Autodesk Inventor part; units mm, degrees
ref_plane "IDS_WORKPLANE{1}" through (-2.8448, 0, 0) normal (1, 0, 0) x (0, 0, -1)
ref_plane "Work Plane2" through (-1.4224, 0, 0) normal (0, 0, -1) x (1, 0, 0)
ref_plane "YZ Plane" through (0, 0, 0) normal (1, 0, 0) x (0, 1, 0)
sketch "Sketch1" plane through (0, 0, 0) normal (0, 0, 1) x (1, 0, 0)
  line L0 (-2.8448, 0) -> (9.525, 0)
  line L1 (9.525, 0) -> (9.525, 1.4224)
  line L2 (9.525, 1.4224) -> (0, 1.4224)
  line L3 (0, 1.4224) -> (0, 2.3241)
  line L4 (-7.3162, 0) -> (16.036, 0)
  line L5 (0, -0.4648) -> (0, 2.7889)
  line L6 (0, 2.3241) -> (-2.8448, 2.3241)
  line L7 (-2.8448, 0) -> (-2.8448, 2.3241)
  arc A0 (-1.1734, 0) -> (-1.5494, 1.4034) centre (-3.9802, 0) ccw
  line L8 (-2.8448, 1.4034) -> (-1.5494, 1.4034)
  line L9 (12.7, 1.4224) -> (0, 1.4224) construction
  dimension "d0" = 9.525
  dimension "d1" = 2.8448
  dimension "d2" = 2.8448
  dimension "d5" = 4.6482
  dimension "d13" = 2.8068
  dimension "d14" = 2.8068
  dimension "d15" = 1.2954
revolve "Body" add sketch "Sketch1" angle 360 about axis through (-2.8448, 0, 0) along (1, 0, 0) contours A0 L8 L7 L6 L3 L5 L0 | L5 L2 L1 L0
ref_plane "IDS_WORKPLANE{1}" through (-2.8448, 0, 0) normal (1, 0, 0) x (0, 0, -1)
sketch "Sketch2" plane through (-2.8448, 0, 0) normal (1, 0, 0) x (0, 0, -1)
  line L0 (0, -3.6027) -> (0, 5.3473)
  line L1 (5.6384, 0) -> (-3.6512, 0)
  circle A0 centre (0, 0) radius 2.3241
  line L2 (1.3655, 0.3238) -> (1.1714, 0.3239)
  line L3 (0, 0) -> (1.3655, 0.3238) construction
  line L4 (0, 0) -> (4.3113, 4.0687) construction
  line L5 (0, 0) -> (0.4023, 1.3445) construction
  line L6 (0, 0) -> (0.7017, 1.2154) construction
  line L7 (0.4023, 1.3445) -> (0.3053, 1.1764)
  line L8 (0.9632, 1.0207) -> (0.8662, 0.8526)
  line L9 (0, 0) -> (0.9632, 1.0207) construction
  arc A1 (1.2154, 0) -> (1.1714, 0.3239) centre (0, 0) ccw
  arc A2 (0.8662, 0.8526) -> (0.3053, 1.1764) centre (0, 0) ccw
  arc A3 (1.4034, 0) -> (1.3655, 0.3238) centre (0, 0) ccw
  arc A4 (0.9632, 1.0207) -> (0.4023, 1.3445) centre (0, 0) ccw
  arc A5 (1.3655, 0.3238) -> (0.8276, 1.1334) centre (0, 0) ccw construction
  arc A6 (1.1714, 0.3239) -> (0.8662, 0.8526) centre (0, 0) ccw construction
  line L10 (1.3655, -0.3238) -> (1.1714, -0.3239)
  line L11 (0.4023, -1.3445) -> (0.3053, -1.1764)
  line L12 (0.9632, -1.0207) -> (0.8662, -0.8526)
  arc A7 (1.1714, -0.3239) -> (1.2154, 0) centre (0, 0) ccw
  arc A8 (0.3053, -1.1764) -> (0.8662, -0.8526) centre (0, 0) ccw
  arc A9 (1.3655, -0.3238) -> (1.4034, 0) centre (0, 0) ccw
  arc A10 (0.4023, -1.3445) -> (0.9632, -1.0207) centre (0, 0) ccw
  line L13 (-1.3655, 0.3238) -> (-1.1714, 0.3239)
  line L14 (-0.4023, 1.3445) -> (-0.3053, 1.1764)
  line L15 (-0.9632, 1.0207) -> (-0.8662, 0.8526)
  arc A11 (-1.1714, 0.3239) -> (-1.2154, 0) centre (0, 0) ccw
  arc A12 (-0.3053, 1.1764) -> (-0.8662, 0.8526) centre (0, 0) ccw
  arc A13 (-1.3655, 0.3238) -> (-1.4034, 0) centre (0, 0) ccw
  arc A14 (-0.4023, 1.3445) -> (-0.9632, 1.0207) centre (0, 0) ccw
  line L16 (-0.4023, -1.3445) -> (-0.3053, -1.1764)
  arc A15 (-0.8662, -0.8526) -> (-0.3053, -1.1764) centre (0, 0) ccw
  line L17 (-0.9632, -1.0207) -> (-0.8662, -0.8526)
  arc A16 (-0.9632, -1.0207) -> (-0.4023, -1.3445) centre (0, 0) ccw
  arc A17 (-1.2154, 0) -> (-1.1714, -0.3239) centre (0, 0) ccw
  line L18 (-1.3655, -0.3238) -> (-1.1714, -0.3239)
  arc A18 (-1.4034, 0) -> (-1.3655, -0.3238) centre (0, 0) ccw
  point P0 (0.7017, -1.2154)
  point P1 (-0.7017, 1.2154)
  point P2 (-0.7017, -1.2154)
  dimension "d19" = 0.3239
  dimension "d20" = 0.6477
  dimension "d21" = 33.316
  dimension "d22" = 2.8068
  dimension "d23" = 2.4308
extrude "Slot" add sketch "Sketch2" along normal up to next contours A1 L2 A3 L1 | L1 A9 L10 A7 | A17 L18 A18 L1 | L1 A13 L13 A11 | A4 L8 A2 L7 | L11 A8 L12 A10 | L14 A12 L15 A14 | A16 L17 A15 L16
fillet "Fillet1" radius 0.2286 1 edges at (-2.8448, -2.3241, 0)
thread "Thread"
chamfer "Chamfer1" distance 0.3785 distance2 0.3785 1 edges at (9.525, -1.4224, 0) measured on face at (9.525, -0.2537, -0.5191)
ref_plane "Work Plane2" through (-1.4224, 0, 0) normal (0, 0, -1) x (1, 0, 0)
equation "\"d19\" = 0.5 * SBR"
equation "\"d20\" = SBR"
equation "\"d22\" = 1.1547 * SW"
equation "\"d23\" = SW"
equation "\"d17\" = INTI"
equation "\"d24\" = RR"
equation "\"d6\" = GEL"
equation "\"d9\" = -0.5 * SPD + 0.5 * NND"
equation "\"d10\" = GUL"
equation "\"d0\" = NLG"
equation "\"d1\" = KOH"
equation "\"d2\" = NND"
equation "\"d5\" = KOD"
equation "\"d13\" = 1.1547 * SW"
equation "\"d14\" = 1.1547 * SW"
equation "\"d15\" = INTI"
equation "\"NND\" = 2.8448"
equation "\"NLG\" = 9.525"
equation "\"GEL\" = 7.9375"
equation "\"KOD\" = 4.6482"
equation "\"KOH\" = 2.8448"
equation "\"SPD\" = GD1"
equation "\"GUL\" = 0.37846"
equation "\"SBR\" = 0.6477"
equation "\"INTI\" = 1.2954"
equation "\"d11\" = -KOH"
equation "\"SW\" = 2.43078"
equation "\"d16\" = 1.1547 * SW"
equation "\"d18\" = SW"
equation "\"RR\" = 0.2286"
equation "\"TOA\" = 30deg"
equation "\"GD1\" = 2.08788"
equation "\"THREADDIA\" = 2.8448"
equation "\"BDM\" = NND"
equation "\"GD\" = NND"
equation "\"GAL\" = 1.5875"
equation "\"E0\" = 2.86258"
properties part number "ANSI B18.3 - 4-40 UNC - 0.375, SSHCSI" material "Steel, Mild"
Design review of the part built by this model. Coordinates are the model's own, in mm. A direction names the side the tool comes from. Give positions to 0.01 mm unless a question says otherwise; leave off trailing zeros. Order: outer loops, then holes, each group sorted by start corner. A loop starts at its lowest first (then second) coordinate and runs counter-clockwise, first axis right, second up. Notation, with made-up numbers: (2.25, 74) - (32.25, 74) arc R36 ccw to (32.25, 111) - close; hole circle Ø8 at (-35.75, -6). An arc over 180 degrees is marked (long way). Use a Markdown table: item, result. Add a question column.
(1) Machinability: for faces 5 (the face through (4.51, -0.31, 1.39)), 6 (the face through (9.525, 0, 0)), which of the approach directions +Z, -Z, +X, -X, +Y, -Y give a long, thin tool a straight path to every point of the face, cutting with its end or side? Answer none if there is none.
(2) Add section A-A on x = 0.25. Give the boundary of the cut face in (y, z).
(3) Clearance check with flat-ended pins moving along their axes: P1, Ø1.5, axis at x = 1.5, z = -1.5, coming from the +Y side; P2, Ø1.5, axis at x = 8, z = 2, coming from the -Y side. State where each tip first meets the part, or that it passes through.
(4) Wall thickness on probe 1 along X at (y, z) = (1.75, -1); probe 2 along Y at (x, z) = (1.75, -0.4) (3 decimals); probe 3 along Z at (x, y) = (5, 0.8): over which ranges is each line inside the solid? List them lowest first. Write a range as [from, to].
(5) Mouldability with a two-part tool opening along Z and no side actions: class faces 1 (the face through (-1.33, -0.5, 2.27)), 2 (the face through (-2.188, -1.403, 0.006)), 3 (the face through (-2.845, 0, -1.4)), 4 (the face through (-2.188, 1.403, -0.006)) as +Z half, -Z half, draft (parallel to the pull), parting line (faces both ways), or undercut.
Report:
| question | item | result |
|---|---|---|
| 1 | face 5 | +X |
| 1 | face 6 | +Z, -Z, +X, +Y, -Y |
| 2 | outline | circle Ø2.84 at (0, 0) |
| 3 | P1 | stops at y = 1.21 |
| 3 | P2 | stops at y = -0.68 |
| 4 | probe 1 | x = [-2.84, 0] |
| 4 | probe 2 | y = [-1.365, 1.365] |
| 4 | probe 3 | z = [-1.18, 1.18] |
| 5 | face 1 | parting line |
| 5 | face 2 | undercut |
| 5 | face 3 | draft |
| 5 | face 4 | undercut |
